from build123d import *

# Parameters (mm, degrees)
F1_DEPTH = 6.35


with BuildPart() as f1:
    # F0 (on Top) → F1 (new body)
    with BuildSketch(Plane.XY):
        with BuildLine():
            Line((-103.585208, 203.2), (-128.985208, 203.2))
            Line((-128.985208, 203.2), (-128.985208, 177.8))
            Line((-128.985208, 177.8), (-124.222708, 177.8))
            ThreePointArc((-124.222708, 177.8), (-122.635208, 179.3875), (-121.047708, 177.8))
            ThreePointArc((-121.047708, 177.8), (-121.512676, 176.677468), (-122.635208, 176.2125))
            Line((-122.635208, 176.2125), (-122.635208, 153.9875))
            ThreePointArc((-122.635208, 153.9875), (-121.512676, 153.522532), (-121.047708, 152.4))
            ThreePointArc((-121.047708, 152.4), (-122.635208, 150.8125), (-124.222708, 152.4))
            Line((-124.222708, 152.4), (-128.985208, 152.4))
            Line((-128.985208, 152.4), (-128.985208, 101.6))
            Line((-128.985208, 101.6), (-124.222708, 101.6))
            ThreePointArc((-124.222708, 101.6), (-122.635208, 103.1875), (-121.047708, 101.6))
            ThreePointArc((-121.047708, 101.6), (-121.512676, 100.477468), (-122.635208, 100.0125))
            Line((-122.635208, 100.0125), (-122.635208, 77.7875))
            ThreePointArc((-122.635208, 77.7875), (-121.512676, 77.322532), (-121.047708, 76.2))
            ThreePointArc((-121.047708, 76.2), (-122.635208, 74.6125), (-124.222708, 76.2))
            Line((-124.222708, 76.2), (-128.985208, 76.2))
            Line((-128.985208, 76.2), (-128.985208, 25.4))
            Line((-128.985208, 25.4), (-124.222708, 25.4))
            ThreePointArc((-124.222708, 25.4), (-122.635208, 26.9875), (-121.047708, 25.4))
            ThreePointArc((-121.047708, 25.4), (-121.512676, 24.277468), (-122.635208, 23.8125))
            Line((-122.635208, 23.8125), (-122.635208, 1.5875))
            ThreePointArc((-122.635208, 1.5875), (-121.512676, 1.122532), (-121.047708, 0))
            ThreePointArc((-121.047708, 0), (-122.635208, -1.5875), (-124.222708, 0))
            Line((-124.222708, 0), (-128.985208, 0))
            Line((-128.985208, 0), (-128.985208, -50.8))
            Line((-128.985208, -50.8), (-124.222708, -50.8))
            ThreePointArc((-124.222708, -50.8), (-122.635208, -49.2125), (-121.047708, -50.8))
            ThreePointArc((-121.047708, -50.8), (-121.512676, -51.922532), (-122.635208, -52.3875))
            Line((-122.635208, -52.3875), (-122.635208, -74.6125))
            ThreePointArc((-122.635208, -74.6125), (-121.512676, -75.077468), (-121.047708, -76.2))
            ThreePointArc((-121.047708, -76.2), (-122.635208, -77.7875), (-124.222708, -76.2))
            Line((-124.222708, -76.2), (-128.985208, -76.2))
            Line((-128.985208, -76.2), (-128.985208, -114.3))
            Line((-128.985208, -114.3), (125.014792, -114.3))
            Line((125.014792, -114.3), (125.014792, -76.2))
            Line((125.014792, -76.2), (120.252292, -76.2))
            ThreePointArc((120.252292, -76.2), (117.54226, -77.322532), (118.664792, -74.6125))
            Line((118.664792, -74.6125), (118.664792, -52.3875))
            ThreePointArc((118.664792, -52.3875), (117.54226, -49.677468), (120.252292, -50.8))
            Line((120.252292, -50.8), (125.014792, -50.8))
            Line((125.014792, -50.8), (125.014792, 0))
            Line((125.014792, 0), (120.252292, 0))
            ThreePointArc((120.252292, 0), (117.54226, -1.122532), (118.664792, 1.5875))
            Line((118.664792, 1.5875), (118.664792, 23.8125))
            ThreePointArc((118.664792, 23.8125), (117.54226, 26.522532), (120.252292, 25.4))
            Line((120.252292, 25.4), (125.014792, 25.4))
            Line((125.014792, 25.4), (125.014792, 76.2))
            Line((125.014792, 76.2), (120.252292, 76.2))
            ThreePointArc((120.252292, 76.2), (117.54226, 75.077468), (118.664792, 77.7875))
            Line((118.664792, 77.7875), (118.664792, 100.0125))
            ThreePointArc((118.664792, 100.0125), (117.54226, 102.722532), (120.252292, 101.6))
            Line((120.252292, 101.6), (125.014792, 101.6))
            Line((125.014792, 101.6), (125.014792, 152.4))
            Line((125.014792, 152.4), (120.252292, 152.4))
            ThreePointArc((120.252292, 152.4), (117.54226, 151.277468), (118.664792, 153.9875))
            Line((118.664792, 153.9875), (118.664792, 176.2125))
            ThreePointArc((118.664792, 176.2125), (117.54226, 178.922532), (120.252292, 177.8))
            Line((120.252292, 177.8), (125.014792, 177.8))
            Line((125.014792, 177.8), (125.014792, 203.2))
            Line((125.014792, 203.2), (99.614792, 203.2))
            Line((99.614792, 203.2), (99.614792, 198.4375))
            ThreePointArc((99.614792, 198.4375), (100.737324, 197.972532), (101.202292, 196.85))
            ThreePointArc((101.202292, 196.85), (99.614792, 195.2625), (98.027292, 196.85))
            Line((98.027292, 196.85), (75.802292, 196.85))
            ThreePointArc((75.802292, 196.85), (73.09226, 195.727468), (74.214792, 198.4375))
            Line((74.214792, 198.4375), (74.214792, 203.2))
            Line((74.214792, 203.2), (20.239792, 203.2))
            Line((20.239792, 203.2), (20.239792, 198.4375))
            ThreePointArc((20.239792, 198.4375), (21.362324, 197.972532), (21.827292, 196.85))
            ThreePointArc((21.827292, 196.85), (20.239792, 195.2625), (18.652292, 196.85))
            Line((18.652292, 196.85), (-22.622708, 196.85))
            ThreePointArc((-22.622708, 196.85), (-25.33274, 195.727468), (-24.210208, 198.4375))
            Line((-24.210208, 198.4375), (-24.210208, 203.2))
            Line((-24.210208, 203.2), (-78.185208, 203.2))
            Line((-78.185208, 203.2), (-78.185208, 198.4375))
            ThreePointArc((-78.185208, 198.4375), (-77.062676, 197.972532), (-76.597708, 196.85))
            ThreePointArc((-76.597708, 196.85), (-78.185208, 195.2625), (-79.772708, 196.85))
            Line((-79.772708, 196.85), (-101.997708, 196.85))
            ThreePointArc((-101.997708, 196.85), (-104.70774, 195.727468), (-103.585208, 198.4375))
            Line((-103.585208, 198.4375), (-103.585208, 203.2))
        make_face()
    extrude(amount=F1_DEPTH)


solid = f1.part
Design review of the part built by this model. Coordinates are the model's own, in mm. A direction names the side the tool comes from. Round coordinates to 2 decimals unless told otherwise and drop trailing zeros. Return JSON: item names as keys, results as strings. Group by question number.
Item 1: Machinability: for faces 1 (the face through (-91, 196.85, 3)), 2 (the face through (-122.635, 13, 3)), 3 (the face through (118.665, 165, 3)), 4 (the face through (-4, 47, 0)), which of the approach directions +Z, -Z, +X, -X, +Y, -Y give a long, thin tool a straight path to every point of the face, cutting with its end or side? Answer none if there is none.
Item 2: For probe 1 along Y at (x, z) = (5.5, 5); probe 2 along X at (y, z) = (-64.5, 4.25); probe 3 along Y at (x, z) = (101, 1.25), list the stretches that pass through material, from the lowest coordinate up. Write a range as [from, to].
Item 3: The part is to be moulded in two halves that separate along X. For faces 5 (the face through (-128.985, -95, 3)), 6 (the face through (87, 196.85, 3)), 7 (the face through (-4, -114.3, 3)), say which applies: pulls with the +X half, pulls with the -X half, needs draft (parallel to the pull), parting line crosses it, or undercut.
Item 4: Insertion check: P1, Ø6, axis at x = 58, y = -74.5, coming from the -Z side; P2, Ø1.9, axis at y = 16.5, z = 4.5, coming from the +X side; P3, Ø3, axis at y = 170, z = 1.5, coming from the -X side; P4, Ø1.9, axis at x = -88.5, z = 4.5, coming from the +Y side. Each pin has a flat end and moves straight along its axis. Give the tip position at first contact, or say it passes through.
Model answer:
{
 "1": {"face 1": "+Z, -Z, +Y", "face 2": "+Z, -Z, -X", "face 3": "+Z, -Z, +X", "face 4": "-Z, +X, -X, +Y, -Y"},
 "2": {"probe 1": "y = [-114.3, 196.85]", "probe 2": "x = [-122.64, 118.66]", "probe 3": "y = [-114.3, 196.07], [197.63, 203.2]"},
 "3": {"face 5": "pulls with the -X half", "face 6": "undercut", "face 7": "needs draft"},
 "4": {"P1": "stops at z = 0", "P2": "stops at x = 118.66", "P3": "stops at x = -122.64", "P4": "stops at y = 196.85"}
}
